Autodesk Inventor part; units mm, degrees
ref_plane "YZ Plane" through (0, 0, 0) normal (1, 0, 0) x (0, 1, 0)
ref_plane "XZ Plane" through (0, 0, 0) normal (0, 1, 0) x (-1, 0, 0)
ref_plane "XY Plane" through (0, 0, 0) normal (0, 0, 1) x (1, 0, 0)
sketch "Sketch1" plane through (0, 0, 0) normal (1, 0, 0) x (0, 1, 0)
  circle A0 centre (4.2685, -9.9057) radius 2.1844
  circle A1 centre (13.7537, 1.1357) radius 2.1844
  circle A2 centre (-9.6373, 11.0363) radius 2.1844
  arc A3 (18.5704, -3.0021) -> (16.2288, 6.9834) centre (13.7537, 1.1357) ccw
  arc A4 (-1.0214, -13.4183) -> (9.0853, -14.0435) centre (4.2685, -9.9057) ccw
  arc A5 (-7.1621, 16.884) -> (-14.9273, 7.5236) centre (-9.6373, 11.0363) ccw
  line L0 (-7.1621, 16.884) -> (16.2288, 6.9834)
  line L1 (-14.9273, 7.5236) -> (-1.0214, -13.4183)
  line L2 (18.5704, -3.0021) -> (9.0853, -14.0435)
  point P0 (0, 0)
  dimension "d0" = 12.7
  dimension "d1" = 12.7
  dimension "d2" = 12.7
extrude "Extrusion1" add sketch "Sketch1" along normal blind 1.5875
properties part number "Conveyer Gusset" material "Acetal Resin, White"
CAD build for the part. Positions are in the model's coordinates, mm. Round coordinates to 2 decimals unless told otherwise and drop trailing zeros. Write each loop counter-clockwise with the first axis right and the second up, starting at its lowest first coordinate (ties: lowest second). Pieces come first, ordered by that corner, then holes. Notation, with made-up numbers: (87, 60.25) -> (124, 60.25) arc R9 cw to (124, 70.25) -> close; hole circle Ø3 at (15, -35.5). An arc over 180 degrees is marked (long way). Answer as a JSON object with one key per item and string values.
(1) Probe probe 1 along Y at (x, z) = (1.3, -11.5); probe 2 along Z at (x, y) = (1.45, -8); probe 3 along Y at (x, z) = (1, -9). List the from-to ranges inside material, lowest first. Write a range as [from, to].
Reported:
{"probe 1": "y = [-2.3, 2.78], [5.76, 11.27]", "probe 2": "z = [-2.91, 9.59], [12.48, 17.17]", "probe 3": "y = [-3.96, 2.28], [6.26, 13.42]"}
(2) Band-saw the part on A-A, the plane z = 10. List the corners of the cut face in (x, y), then the cut area to 3 significant figures.
Reported:
{"outline": "(0, -15.9) -> (1.59, -15.9) -> (1.59, -11.56) -> (0, -11.56) -> close; (0, -7.71) -> (1.59, -7.71) -> (1.59, 9.1) -> (0, 9.1) -> close", "area": "33.6 mm^2"}
(3) Two-plate mould, pull along Y, no slides. Class faces 1 (the face through (0, 2, 1)), 2 (the face through (0.78, -11.25, 9.56)), 3 (the face through (0.783, 4.37, 12.003)): +Y half, -Y half, draft (parallel to the pull), parting line (faces both ways), or undercut.
Reported:
{"face 1": "draft", "face 2": "undercut", "face 3": "+Y half"}
(4) Band-saw the part on B-B, the plane y = -11. List the corners of the cut face in (x, z).
Reported:
{"outline": "(0, 1.61) -> (1.59, 1.61) -> (1.59, 9.33) -> (0, 9.33) -> close; (0, 12.74) -> (1.59, 12.74) -> (1.59, 17.24) -> (0, 17.24) -> close"}
(5) Band-saw the part on D-D, the plane y = 7.5. List the corners of the cut face in (x, z).
Reported:
{"outline": "(0, -15.37) -> (1.59, -15.37) -> (1.59, 10.68) -> (0, 10.68) -> close"}
(6) Band-saw the part on C-C, the plane x = 0.9. List the corners of the cut face in (y, z).
Reported:
{"outline": "(-14.93, 7.52) -> (-1.02, -13.42) arc R6.35 ccw to (9.09, -14.04) -> (18.57, -3) arc R6.35 ccw to (16.23, 6.98) -> (-7.16, 16.88) arc R6.35 ccw to start; hole circle Ø4.37 at (-9.64, 11.04); hole circle Ø4.37 at (4.27, -9.91); hole circle Ø4.37 at (13.75, 1.14)"}
